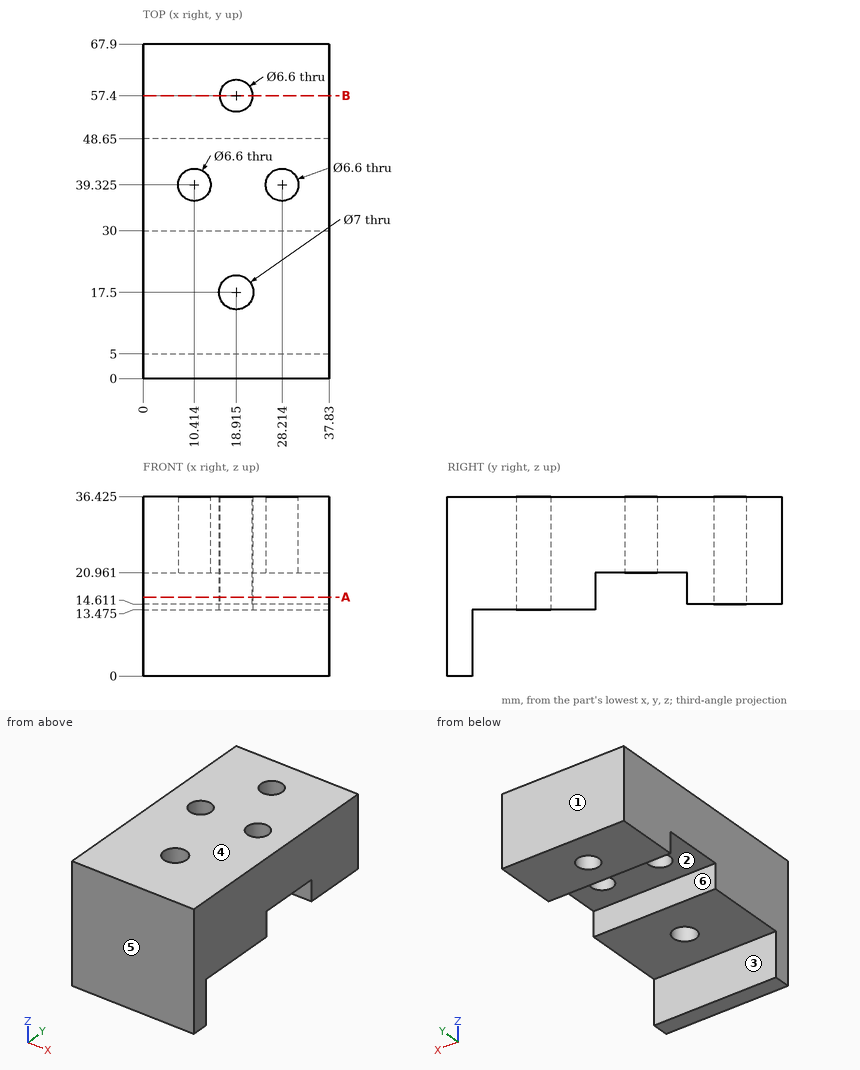
For this review, use the dimensioned drawing (mm, ordinates from the lowest corner) and the shaded views. A direction names the side the tool comes from. Round coordinates to 2 decimals unless told otherwise and drop trailing zeros. Order: outer loops, then holes, each group sorted by start corner. A loop starts at its lowest first (then second) coordinate and runs counter-clockwise, first axis right, second up. Notation, with made-up numbers: M -14.75,13.25 L 38.25,13.25 A13 cw 38.25,28.25 Z; hole C 3.25,4 d4. An arc over 180 degrees is marked long. Use a Markdown table: item, result. Add a question column.
Item 1: Add section A-A, the plane z = 16. State how many separate pieces and enclosed holes the cut face has, then the cut area to 3 significant figures.
Item 2: Mouldability with a two-part tool opening along Y and no side actions: class the marked faces 4, 5 and 6 as released by +Y, released by -Y, zero draft, split by the parting line, or undercut.
Item 3: Add section B-B, the plane y = 57.4. Give the boundary of the cut face in (x, z) (1 decimal).
Item 4: Tool access review of the marked faces 1, 2 and 3: name each direction out of +Z, -Z, +X, -X, +Y, -Y from which nothing blocks a thin tool from reaching the whole face with its end or side.
Item 5: Insertion check: pin 1 (2 mm diameter, centred on x = 31, z = 4, fed in from +Y); pin 2 (1.5 mm diameter, centred on x = 7.5, y = 7, fed in from -Z) (1 decimal); pin 3 (8.5 mm diameter, centred on x = 10.41, y = 39.33, fed in from -Z). Each pin has a flat end and moves straight along its axis. Give the tip position at first contact, or say it passes through.
Item 6: To check wall thickness, follow line 1 along Y through (x, z) = (31, 17); line 2 along Y through (x, z) = (28, 32); line 3 along X through (y, z) = (40, 27) (1 decimal). State the ranges of each line that lie inside material, in increasing order.
Geometry results:
| question | item | result |
|---|---|---|
| 1 | separate pieces | 2 |
| 1 | enclosed holes | 2 |
| 1 | area | 1,790 mm² |
| 2 | face 4 | zero draft |
| 2 | face 5 | released by -Y |
| 2 | face 6 | undercut |
| 3 | outline | M 0,14.6 L 15.6,14.6 L 15.6,36.4 L 0,36.4 Z; M 22.2,14.6 L 37.8,14.6 L 37.8,36.4 L 22.2,36.4 Z |
| 4 | face 1 | +Z, -Z, +X, -X, +Y |
| 4 | face 2 | -Z, +X, -X |
| 4 | face 3 | -Z, +X, -X, +Y |
| 5 | pin 1 | stops at y = 5 |
| 5 | pin 2 | stops at z = 13.5 |
| 5 | pin 3 | stops at z = 20.96 |
| 6 | line 1 | y = 0 to 30, 48.65 to 67.9 |
| 6 | line 2 | y = 0 to 36.03, 42.62 to 67.9 |
| 6 | line 3 | x = 0 to 7.2, 13.6 to 25, 31.4 to 37.8 |
